Could you check a few things on this model? Use its own coordinates, in mm. Coordinates: 2 decimals unless noted, no trailing zeros. Write each loop counter-clockwise with the first axis right and the second up, starting at its lowest first coordinate (ties: lowest second). Pieces come first, ordered by that corner, then holes. Notation, with made-up numbers: (34, 47) - (79, 47) arc R21 cw to (79, 79) - close; hole circle Ø4 at (12.25, 80.5). An arc over 180 degrees is marked (long way). Write item = value, one per line. Start each with the question number.
```python
from build123d import *

# Parameters (mm, degrees)
BOSS_EXTRUDE1_DEPTH = 75
FILLET1_R           = 10


# Read off the part's stored shape, not the designer's step: Boss-Extrude1
with BuildPart() as part:
    # Boss-Extrude1 outline → Boss-Extrude1 (new body)
    with BuildSketch(Plane(origin=(0, 0, 0), x_dir=(1, 0, 0), z_dir=(0, 1, 0))):
        with BuildLine():
            ThreePointArc((179.220822611, 43.207097385), (164.591443385, 76.212397447), (128.83092118, 71.25723646))
            ThreePointArc((128.83092118, 71.25723646), (80.227844704, 46.271602396), (26.129473888, 54.011578336))
            ThreePointArc((26.129473888, 54.011578336), (-53.844334239, 26.472394497), (-26.8142447, -53.674912959))
            ThreePointArc((-26.8142447, -53.674912959), (99.687960456, -55.177812298), (179.220822611, 43.207097385))
        make_face()
    extrude(amount=BOSS_EXTRUDE1_DEPTH)

    # Fillet1
    fillet1_edges = [part.edges().sort_by_distance(p)[0] for p in [
        (99.687960456, 75, 55.177812298),
        (164.591443385, 75, -76.212397447),
        (80.227844704, 75, -46.271602396),
        (-53.844334239, 75, -26.472394497),
    ]]
    fillet(fillet1_edges, radius=FILLET1_R)


solid = part.part
```
1) If I drill on probe 1 along Z at (x, y) = (-48, 25); probe 2 along Z at (x, y) = (23, 15); probe 3 along X at (y, z) = (38, -37), over which ranges is the centre line in solid material (lowest first)? Write a range as [from, to].
2) For P1, Ø4, axis at y = 12.5, z = -54, coming from the +X side; P2, Ø2, axis at y = 11.5, z = -13.5, coming from the +X side; P3, Ø8, axis at y = 25, z = -14.5, coming from the -X side, each with a flat end and sliding along its axis, tell me the tip position at first contact or that it passes through.
3) Suppose I cut it at A-A on y = 19.5. Please give me the cut outline in (x, z), plus the area to 3 significant figures.
4) Thinking about a two-plate mould opening in X: for faces 1 (the cylindrical face through (98.02, 32.04, 55.95)), 2 (the cylindrical face through (80.994, 32.045, -46.404)), 3 (the flat face through (58, 75, -6)), which applies, +X half, -X half, draft (parallel to the pull), parting line (faces both ways), or undercut?
Reply:
q1.probe_1 = [-36, 36]
q1.probe_2 = [-55.42, 68.18]
q1.probe_3 = [-47.23, 177.63]
q2.P1 = 179.93
q2.P2 = 169.28
q2.P3 = -59.07
q3.outline = (-26.81, 53.67) arc R60 ccw to (26.13, -54.01) arc R90 cw to (128.83, -71.26) arc R30 ccw to (179.22, -43.21) arc R145 ccw to start
q3.area = 24,500 mm^2
q4.face_1 = parting line
q4.face_2 = undercut
q4.face_3 = draft
